from build123d import *

# Parameters (mm, degrees)
MODEL_W             = 6.88
MODEL_H             = 15
BOSS_EXTRUDE1_DEPTH = 6.6


with BuildPart() as part:
    # Model → Boss-Extrude1 (new body)
    with BuildSketch(Plane.XY):
        with BuildLine():
            Line((0, -59.622366364), (-4, -59.622366364))
            ThreePointArc((-4, -59.622366364), (-5.767766953, -58.890133317), (-6.5, -57.122366364))
            Line((-6.5, -57.122366364), (-6.5, -37.122366364))
            ThreePointArc((-6.5, -37.122366364), (-5.767766953, -35.354599411), (-4, -34.622366364))
            Line((-4, -34.622366364), (0, -34.622366364))
            Line((0, -34.622366364), (0, -6.035533906))
            ThreePointArc((0, -6.035533906), (1.543291419, -3.725835075), (4.267766953, -4.267766953))
            Line((4.267766953, -4.267766953), (57.275649276, -57.275649276))
            Line((57.275649276, -57.275649276), (59.446467094, -55.104831458))
            Line((59.446467094, -55.104831458), (61.214234047, -56.872598411))
            ThreePointArc((61.214234047, -56.872598411), (61.946467094, -58.640365364), (61.214234047, -60.408132317))
            Line((61.214234047, -60.408132317), (50.732233047, -70.890133317))
            ThreePointArc((50.732233047, -70.890133317), (49.921174675, -71.432065195), (48.964466094, -71.622366364))
            Line((48.964466094, -71.622366364), (24.482233047, -71.622366364))
            Line((24.482233047, -71.622366364), (3.651186429, -82.428337026))
            ThreePointArc((3.651186429, -82.428337026), (1.201532841, -82.345502849), (0, -80.209154788))
            Line((0, -80.209154788), (0, -59.622366364))
        make_face()
        with Locations((3.44, -47.122366364)):
            Rectangle(MODEL_W, MODEL_H, mode=Mode.SUBTRACT)
    extrude(amount=BOSS_EXTRUDE1_DEPTH)


solid = part.part
Input: part model. Units: mm. Frame: model coordinates. A direction names the side the tool comes from. Coordinates: 2 decimals unless noted, no trailing zeros. Loops run counter-clockwise (first coordinate to the right, second up) from the corner with the lowest first, then second, coordinate; pieces in that order, holes last.
(1) Section A-A on y = -51.5. Return the cut outline in (x, z).
(2) Material intervals for probe 1 along Y at (x, z) = (0.5, 5.5); probe 2 along Y at (x, z) = (-3, 5); probe 3 along Y at (x, z) = (5, 4.5), sorted ascending.
(3) Section B-B on z = 1. Return the cut outline in (x, y).
(4) Pull-direction query (Y, two-part tool) for faces 1 (the face through (3, -54.622, 3)), 2 (the face through (0, -70, 3)), 3 (the face through (1.232, -82.364, 3.254)), 4 (the face through (30, -30, 3)); classes: released by +Y, released by -Y, zero draft, split by the parting line, or undercut.
(5) Section C-C on x = 38. Return the cut outline in (y, z).
(6) Section D-D on x = 31. Return the cut outline in (y, z).
(7) First-contact query: pin 1 Ø3.5 at (y, z) = (-49, 2) entering from +X; pin 2 Ø3 at (x, z) = (-3, 2.5) entering from +Y; pin 3 Ø2 at (y, z) = (-73, 4.5) entering from -X. Flat tips, straight axial feed; report the tip coordinate or a pass-through.
(8) Set-up query: faces 5 (the face through (37, -71.622, 3)), 6 (the face through (0, -21, 3)), 7 (the face through (6.88, -47, 3)), 8 (the face through (21, -51, 0)), 9 (the face through (58.346, -56.205, 3.254)). Return all of +Z, -Z, +X, -X, +Y, -Y with unobstructed straight access to the full face (end or side cutting, diameter ignored); none if empty.
Data:
1. outline: (-6.5, 0) - (0, 0) - (0, 6.6) - (-6.5, 6.6) - close; (6.88, 0) - (51.5, 0) - (51.5, 6.6) - (6.88, 6.6) - close
2. probe 1: y = -81.71 to -54.62, -39.62 to -4.54
2. probe 2: y = -59.62 to -34.62
2. probe 3: y = -81.73 to -54.62, -39.62 to -5
3. outline: (-6.5, -57.12) arc R2.5 ccw to (-4, -59.62) - (0, -59.62) - (0, -80.21) arc R2.5 ccw to (3.65, -82.43) - (24.48, -71.62) - (48.96, -71.62) arc R2.5 ccw to (50.73, -70.89) - (61.21, -60.41) arc R2.5 ccw to (61.21, -56.87) - (59.45, -55.1) - (57.28, -57.28) - (4.27, -4.27) arc R2.5 ccw to (0, -6.04) - (0, -34.62) - (-4, -34.62) arc R2.5 ccw to (-6.5, -37.12) - close; hole (0, -54.62) - (6.88, -54.62) - (6.88, -39.62) - (0, -39.62) - close
4. face 1: undercut
4. face 2: zero draft
4. face 3: released by -Y
4. face 4: released by +Y
5. outline: (-71.62, 0) - (-38, 0) - (-38, 6.6) - (-71.62, 6.6) - close
6. outline: (-71.62, 0) - (-31, 0) - (-31, 6.6) - (-71.62, 6.6) - close
7. pin 1: stops at x = 50.75
7. pin 2: stops at y = -34.62
7. pin 3: stops at x = 0
8. face 5: +Z, -Z, +X, -Y
8. face 6: +Z, -Z, -X, +Y
8. face 7: +Z, -Z
8. face 8: -Z, +X, -X, +Y, -Y
8. face 9: +Z, -Z, +Y
